Autodesk Inventor part; units mm, degrees
ref_plane "YZ Plane" through (0, 0, 0) normal (1, 0, 0) x (0, 1, 0)
ref_plane "XZ Plane" through (0, 0, 0) normal (0, 1, 0) x (-1, 0, 0)
ref_plane "XY Plane" through (0, 0, 0) normal (0, 0, 1) x (1, 0, 0)
sketch "Sketch1" plane through (0, 0, 0) normal (0, 1, 0) x (-1, 0, 0)
  circle A0 centre (-26.1551, -3.0475) radius 2
  arc A1 (-34.9051, -0.0475) -> (-17.4051, -0.0475) centre (-26.1551, -0.0475) ccw
  arc A2 (17.5949, -0.0475) -> (35.0949, -0.0475) centre (26.3449, -0.0475) ccw
  circle A3 centre (26.3449, -3.0475) radius 2
  circle A4 centre (-26.1551, -3.0475) radius 2
  circle A5 centre (26.3449, -3.0475) radius 2
  circle A6 centre (26.3449, -0.0475) radius 8.75
  circle A7 centre (-26.1551, -0.0475) radius 8.75
  line L0 (-34.9051, -0.0475) -> (-17.4051, -0.0475)
  line L1 (17.5949, -0.0475) -> (35.0949, -0.0475)
  circle A8 centre (-26.1551, -3.0475) radius 5.5
  circle A9 centre (26.3449, -3.0475) radius 5.5
  line L2 (-26.1551, -8.5475) -> (26.3449, -8.5475)
  line L3 (-26.1551, 2.4525) -> (26.3449, 2.4525)
  point P0 (0, 0)
  dimension "d0" = 11
  dimension "d1" = 11
extrude "Extrusion1" add sketch "Sketch1" along normal blind 10 contours L2 A8 L0 A1 | A1 A7 L3 A6 A2 L2 | A7 L0 A8 L3 | A8 L0 | L0 A8 | A2 L1 A9 L2 | L3 A9 L1 A6 | A9 L1 | A9 L1 picked at (-18.6939, -1.0014) picked at (-20.5799, 1.133) picked at (18.8536, -1.0809) picked at (20.7697, 1.133)
sketch "Sketch2" plane through (0, 10, 0) normal (0, 1, 0) x (1, 0, 0)
  line L0 (26.1551, 8.5475) -> (-26.3449, 8.5475)
  line L1 (-26.3449, -2.4525) -> (26.1551, -2.4525)
  arc A0 (-26.3449, 8.5475) -> (-26.3449, -2.4525) centre (-26.3449, 3.0475) ccw
  arc A1 (26.1551, -2.4525) -> (26.1551, 8.5475) centre (26.1551, 3.0475) ccw
  line L2 (-31.8449, 3.0475) -> (31.6551, 3.0475)
  line L3 (13.4051, -3.4525) -> (-13.5949, -3.4525)
  line L4 (-13.5949, -3.4525) -> (-13.5949, 9.5475)
  line L5 (-13.5949, 9.5475) -> (13.4051, 9.5475)
  line L6 (13.4051, 9.5475) -> (13.4051, -3.4525)
  line L7 (13.4051, -3.4525) -> (-13.5949, 9.5475) construction
  line L8 (-13.5949, -3.4525) -> (13.4051, 9.5475) construction
  point P0 (0, 0)
  point P1 (-0.0949, 3.0475)
  dimension "d4" = 27
  dimension "d5" = 13
extrude "Extrusion2" add sketch "Sketch2" along normal blind 14.56 contours L6 L2 L4 L0 | L0 L4 L5 L6 | L6 L1 L4 L2 | L6 L3 L4 L1
fillet "Fillet1" radius 2 2 edges at (-0.0949, 10, 3.4525) (-0.0949, 10, -9.5475)
sketch "Sketch3" plane through (0, 24.56, 0) normal (0, 1, 0) x (1, 0, 0)
  arc A0 (-6.3236, 1.0357) -> (-4.0158, 1.1475) centre (-5.0949, -0.4525) ccw
  arc A1 (3.5842, 1.1475) -> (6.0652, 1.2676) centre (4.9051, -0.4525) ccw
  circle A2 centre (4.9051, -0.4525) radius 2.0748
  circle A3 centre (-5.0949, -0.4525) radius 1.9299
  line L0 (-13.5949, 9.5475) -> (-13.5949, -3.4525)
  line L1 (13.4051, 9.5475) -> (-13.5949, 9.5475)
  line L2 (-13.5949, -3.4525) -> (13.4051, -3.4525)
  line L3 (13.4051, -3.4525) -> (13.4051, 9.5475)
  point P0 (0, 0)
  point P1 (6.0652, 1.2676)
  point P2 (-4.0158, 1.1475)
  dimension "d12" = 8.5
  dimension "d13" = 8.5
extrude "Extrusion3" cut sketch "Sketch3" against normal blind 10 contours A3 A0 | A2 A1
sketch "Sketch4" plane through (0, 24.56, 0) normal (0, 1, 0) x (1, 0, 0)
  line L0 (13.4051, 9.5475) -> (-13.5949, 9.5475)
  line L1 (-13.5949, -2.4525) -> (-13.5949, 8.5475)
  line L2 (13.4051, 9.5475) -> (-13.5949, 9.5475)
  line L3 (-13.5949, 9.5475) -> (-13.5949, 3.0475)
  line L4 (-13.5949, 3.0475) -> (13.4051, 3.0475)
  line L5 (13.4051, 3.0475) -> (13.4051, 9.5475)
  point P0 (0, 0)
extrude "Extrusion4" cut sketch "Sketch4" against normal blind 4.2875
fillet "Fillet2" radius 6.7625 1 edges at (-0.0949, 20.2725, -9.5475)
sketch "Sketch5" plane through (0, 24.56, 0) normal (0, 1, 0) x (1, 0, 0)
  line L0 (-13.5949, -3.4525) -> (13.4051, -3.4525)
  line L1 (-10.3949, -3.4525) -> (-10.3949, -67.4525)
  line L2 (10.2051, -3.4525) -> (10.2051, -67.4525)
  line L3 (-13.5949, 3.0475) -> (-13.5949, -3.4525)
  circle A0 centre (-5.0949, -49.4525) radius 2
  line L4 (13.4051, -3.4525) -> (13.4051, 3.0475)
  circle A1 centre (4.9051, -49.4525) radius 2
  circle A2 centre (4.9051, -49.4525) radius 3
  circle A3 centre (-5.0949, -49.4525) radius 3
  line L5 (-10.3949, -67.4525) -> (10.2051, -67.4525)
  line L6 (-10.3949, -67.4525) -> (-13.5949, -67.4525)
  line L7 (-13.5949, -67.4525) -> (-13.5949, -3.4525)
  line L8 (10.2051, -67.4525) -> (13.4051, -67.4525)
  line L9 (13.4051, -67.4525) -> (13.4051, -3.4525)
  line L10 (-5.0949, -46.4525) -> (4.9051, -46.4525)
  line L11 (10.2051, -46.4525) -> (-10.3949, -46.4525)
  line L12 (-0.65, -46.4525) -> (-0.65, -51.4525)
  line L13 (-0.65, -51.4525) -> (0.65, -51.4525)
  line L14 (0.65, -51.4525) -> (0.65, -46.4525)
  line L15 (0, -46.4525) -> (-0.65, -51.4525) construction
  line L16 (0, -46.4525) -> (0.65, -51.4525) construction
  point P0 (0, 0)
  point P1 (13.4051, -0.2025)
  point P2 (4.9051, -46.4525)
  dimension "d28" = 6
  dimension "d29" = 6
  dimension "d19" = 3.2
  dimension "d20" = 64
  dimension "d21" = 3.2
  dimension "d22" = 64
  dimension "d23" = 46
  dimension "d24" = 8.5
  dimension "d25" = 4
  dimension "d26" = 8.5
  dimension "d27" = 4
  dimension "d30" = 1.3
extrude "Extrusion5" add sketch "Sketch5" against normal blind 4.2875 contours L0 L1 L6 L7 | L0 L9 L8 L2 | A2 | A3 | L11 L10 L12 L13 L14 L2 L5 L1
properties part number "Servo_Holder"
Check sheet for the modelled part. Datum: model origin and axes. Units: mm. A direction names the side the tool comes from. Coordinates: 2 decimals unless noted, no trailing zeros. Write each loop counter-clockwise with the first axis right and the second up, starting at its lowest first coordinate (ties: lowest second). Pieces come first, ordered by that corner, then holes. Notation, with made-up numbers: M 34,-18.75 L 41,-18.75 A28 cw 41,-0.75 Z; hole C 73.5,82 d4. An arc over 180 degrees is marked long. Answer as CSV lines item,"result".
Q1. Cross-section at A-A (z = 27.5). Record the boundary of the cut face in (x, y), then the cut area to 3 significant figures.
Check result:
outline,"M -13.59,20.27 L -10.39,20.27 L -10.39,24.56 L -13.59,24.56 Z; M 10.21,20.27 L 13.41,20.27 L 13.41,24.56 L 10.21,24.56 Z"
area,"27.4 mm^2"
Q2. Mould release check, pull along Z, two halves, no side actions. Record for faces 1 (the face through (-31.844, 4.93, -2.927)), 2 (the face through (-28.25, 4.93, -3.65)), 3 (the face through (0, 5, -8.548)): released by +Z, released by -Z, zero draft, split by the parting line, or undercut.
Check result:
face 1,"split by the parting line"
face 2,"undercut"
face 3,"released by -Z"
Q3. Cross-section at C-C (y = 5). Record the boundary of the cut face in (x, z), then the cut area to 3 significant figures.
Check result:
outline,"M -26.34,-8.55 L 26.16,-8.55 A5.5 ccw 26.16,2.45 L -26.34,2.45 A5.5 ccw Z; hole C -26.34,-3.05 d4; hole C 26.16,-3.05 d4"
area,"647 mm^2"
Q4. Cross-section at B-B (x = 27). Record the boundary of the cut face in (y, z), then the cut area to 3 significant figures.
Check result:
outline,"M 0,-8.48 L 10,-8.48 L 10,-4.86 L 0,-4.86 Z; M 0,-1.23 L 10,-1.23 L 10,2.39 L 0,2.39 Z"
area,"72.4 mm^2"
Q5. Go/stop test with flat-tipped pins: pin 1 (4 mm diameter, centred on y = 6.5, z = 1.5, fed in from +X); pin 2 (3 mm diameter, centred on x = -5, z = 0, fed in from +Y); pin 3 (3.5 mm diameter, centred on y = 23, z = 50, fed in from -X); pin 4 (3 mm diameter, centred on x = -13, z = 47, fed in from -Y). Record where each tip stops, or that it passes through.
Check result:
pin 1,"x = 31.03"
pin 2,"y = 24.56"
pin 3,"x = -13.59"
pin 4,"y = 20.27"
Q6. Material ranges on probe 1 along X at (y, z) = (19.5, 0); probe 2 along X at (y, z) = (22.5, 31.5); probe 3 along Z at (x, y) = (-20.5, 7), recorded low to high. Write a range as from..to.
Check result:
probe 1,"-13.59..-6.97, -3.22..2.88, 6.93..13.41"
probe 2,"-13.59..-10.39, 10.21..13.41"
probe 3,"-8.55..2.45"
Q7. Set-up check for faces 4 (the face through (0, 22, -3.048)), 5 (the face through (10.205, 22, 25)), 6 (the face through (-13.595, 22, 29)), 7 (the face through (4.933, 19.63, 2.527)), 8 (the face through (0.09, 10.74, 3.19)): record each of +Z, -Z, +X, -X, +Y, -Y from which the full face is reachable in a straight line by a thin tool's end or side.
Check result:
face 4,"-Z, +X, -X, +Y"
face 5,"+Y, -Y"
face 6,"+Z, -Z, -X, +Y"
face 7,"+Y"
face 8,"+Z, +X, -X, -Y"
Q8. Cross-section at D-D (x = 4.5). Record the boundary of the cut face in (y, z) (1 decimal), then the cut area to 3 significant figures.
Check result:
outline,"M 0,-8.5 L 10,-8.5 A2 ccw 11.7,-9.5 L 13.5,-9.5 A6.8 ccw 20.3,-3 L 24.6,-3 L 24.6,-1.6 L 14.6,-1.6 L 14.6,2.5 L 24.6,2.5 L 24.6,3.5 L 11.7,3.5 A2 ccw 10,2.5 L 0,2.5 Z; M 20.3,46.5 L 24.6,46.5 L 24.6,47.5 L 20.3,47.5 Z; M 20.3,51.4 L 24.6,51.4 L 24.6,67.5 L 20.3,67.5 Z"
area,"293 mm^2"
